Here's how the part is built. I have some questions about the finished solid (model axes, mm). Face numbers are marked on the shaded views. A direction names the side the tool comes from. Give positions to 0.01 mm unless a question says otherwise; leave off trailing zeros. Write each loop counter-clockwise with the first axis right and the second up, starting at its lowest first coordinate (ties: lowest second). Pieces come first, ordered by that corner, then holes. Notation, with made-up numbers: (7, 53.25) -> (21, 53.25) arc R31 cw to (21, 86.25) -> close; hole circle Ø4 at (48.5, 51). An arc over 180 degrees is marked (long way). Return JSON: item names as keys, results as strings.
Autodesk Inventor part; units mm, degrees
ref_plane "YZ Plane" through (0, 0, 0) normal (1, 0, 0) x (0, 1, 0)
ref_plane "XZ Plane" through (0, 0, 0) normal (0, 1, 0) x (-1, 0, 0)
ref_plane "XY Plane" through (0, 0, 0) normal (0, 0, 1) x (1, 0, 0)
sketch "Sketch1" plane through (0, 0, 0) normal (0, 0, 1) x (1, 0, 0)
  line L0 (9.6801, -14.008) -> (7.2052, -11.5331) construction
  line L1 (7.2052, -11.5331) -> (11.5893, -7.1491) construction
  line L2 (11.5893, -7.1491) -> (14.0642, -9.6239) construction
  line L3 (14.0642, -9.6239) -> (9.6801, -14.008) construction
  arc A0 (12.6369, -4.7496) -> (4.7496, -12.6369) centre (0, 0) ccw construction
  line L4 (10.9298, -3.0424) -> (12.6369, -4.7496) construction
  line L5 (11.6618, -4.6122) -> (10.9298, -3.0424) construction
  arc A1 (11.6618, -4.6122) -> (10.8551, -4.47) centre (11.2086, -4.8235) ccw construction
  line L6 (10.7915, -4.5335) -> (10.8551, -4.47) construction
  arc A2 (10.7915, -4.5335) -> (10.6527, -4.9738) centre (11.1451, -4.887) ccw construction
  line L7 (10.915, -6.4612) -> (10.6527, -4.9738) construction
  arc A3 (10.7761, -6.9016) -> (10.915, -6.4612) centre (10.4226, -6.548) ccw construction
  line L8 (6.9016, -10.7761) -> (10.7761, -6.9016) construction
  arc A4 (6.4612, -10.915) -> (6.9016, -10.7761) centre (6.548, -10.4226) ccw construction
  line L9 (6.4612, -10.915) -> (4.9738, -10.6527) construction
  arc A5 (4.9738, -10.6527) -> (4.5335, -10.7915) centre (4.887, -11.1451) ccw construction
  line L10 (4.5335, -10.7915) -> (4.47, -10.8551) construction
  arc A6 (4.47, -10.8551) -> (4.6122, -11.6618) centre (4.8235, -11.2086) ccw construction
  line L11 (4.6122, -11.6618) -> (3.0424, -10.9298) construction
  line L12 (3.0424, -10.9298) -> (4.7496, -12.6369) construction
  line L13 (-1.7167, -14.6498) -> (-1.7167, -17.5) construction
  line L14 (-1.7167, -17.5) -> (1.7167, -17.5) construction
  line L15 (1.7167, -14.6498) -> (1.7167, -17.5) construction
  arc A7 (1.7167, -14.6498) -> (6.9595, -13.0049) centre (0, 0) ccw construction
  arc A8 (6.9595, -13.0049) -> (8.2728, -15.1789) centre (8.2994, -13.6792) ccw construction
  line L16 (8.2728, -15.1789) -> (7.6816, -15.1684) construction
  arc A9 (8.5249, -17.8901) -> (7.6816, -15.1684) centre (7.655, -16.6682) ccw construction
  line L17 (8.5249, -17.8901) -> (13.5161, -14.3366) construction
  line L18 (13.5161, -14.3366) -> (13.5161, -12.2823) construction
  line L19 (13.5161, -12.2823) -> (14.6168, -12.2823) construction
  line L20 (14.6168, -12.2823) -> (14.6168, -1.9776) construction
  arc A10 (14.6168, -1.9776) -> (1.7167, 14.6498) centre (0, 0) ccw construction
  line L21 (1.7167, 14.6498) -> (1.7167, 17.5) construction
  line L22 (-1.7167, 17.5) -> (1.7167, 17.5) construction
  line L23 (-1.7167, 14.6498) -> (-1.7167, 17.5) construction
  arc A11 (-1.7167, 14.6498) -> (-14.2817, -3.6872) centre (0, 0) ccw construction
  line L24 (-14.2817, -3.6872) -> (-15.4135, -5.7935) construction
  arc A12 (-15.4135, -5.7935) -> (-14.5984, -8.502) centre (-13.6517, -6.7402) ccw construction
  line L25 (-14.5984, -8.502) -> (-9.6326, -11.1703) construction
  arc A13 (-9.6326, -11.1703) -> (-1.7167, -14.6498) centre (0, 0) ccw construction
  line L26 (-24.6, 24.6) -> (25.2, -25.2) construction
  line L27 (25.2, 24.6) -> (-24.6, -25.2) construction
  arc A14 (-1.7471, 10.1) -> (-9.6204, -3.5369) centre (0, 0) ccw
  circle A15 centre (0, 0) radius 10.1 construction
  line L28 (-1.7471, 10.1) -> (1.7471, 10.1)
  line L29 (-7.8733, -6.5631) -> (-9.6204, -3.5369)
  line L30 (9.6204, -3.5369) -> (7.8733, -6.5631)
  arc A16 (1.7471, 10.1) -> (-1.7471, 10.1) centre (0, 0) ccw
  arc A17 (9.6204, -3.5369) -> (1.7471, 10.1) centre (0, 0) ccw
  arc A18 (7.8733, -6.5631) -> (9.6204, -3.5369) centre (0, 0) ccw
  arc A19 (-7.8733, -6.5631) -> (7.8733, -6.5631) centre (0, 0) ccw
  arc A20 (-9.6204, -3.5369) -> (-7.8733, -6.5631) centre (0, 0) ccw
  arc A21 (10.7786, -4.5205) -> (10.6704, -4.6789) centre (11.1451, -4.887) ccw construction
  line L31 (10.7786, -4.5205) -> (10.8421, -4.457) construction
  arc A22 (11.7261, -4.7937) -> (10.8421, -4.457) centre (11.2086, -4.8235) ccw construction
  line L32 (11.7261, -4.7937) -> (10.8691, -2.9558) construction
  line L33 (10.8691, -2.9558) -> (12.6297, -4.7164) construction
  line L34 (4.7164, -12.6297) -> (2.9558, -10.8691) construction
  line L35 (2.9558, -10.8691) -> (4.4463, -11.5641) construction
  arc A23 (4.457, -10.8421) -> (4.4463, -11.5641) centre (4.8235, -11.2086) ccw construction
  line L36 (4.457, -10.8421) -> (4.5223, -10.7767) construction
  arc A24 (4.977, -10.6346) -> (4.6789, -10.6704) centre (4.887, -11.1451) ccw
  arc A25 (4.6789, -10.6704) -> (4.5223, -10.7767) centre (4.887, -11.1451) ccw construction
  arc A26 (10.6704, -4.6789) -> (10.6346, -4.977) centre (11.1451, -4.887) ccw
  circle A27 centre (0, 0) radius 12.65
  dimension "d4" = 20.2
  dimension "d6" = 20.5
  dimension "d9" = 360
  dimension "d28" = 25.3
extrude "Extrusion1" add sketch "Sketch1" against normal blind 5 contours A16 L28 | L29 A20 | A18 L30 | A27
sketch "Sketch3" plane through (0, 0, -5) normal (0, 0, -1) x (-1, 0, 0)
  arc A0 (-7.8733, -6.5631) -> (7.8733, -6.5631) centre (0, 0) ccw
  circle A1 centre (0, 0) radius 9
  circle A2 centre (0, 0) radius 11.5312
  circle A3 centre (0, 0) radius 12.65
  line L0 (9.6204, -3.5369) -> (7.8733, -6.5631)
  line L1 (-7.8733, -6.5631) -> (-9.6204, -3.5369)
  arc A4 (-1.7471, 10.1) -> (-9.6204, -3.5369) centre (0, 0) ccw
  line L2 (-1.7471, 10.1) -> (1.7471, 10.1)
  arc A5 (9.6204, -3.5369) -> (1.7471, 10.1) centre (0, 0) ccw
  dimension "d17" = 18
extrude "Extrusion3" add sketch "Sketch3" along normal blind 10 contours L1 A4 L2 A5 L0 A0 | A2 | A3
sketch "Sketch4" plane through (0, -10.7054, 0) normal (1, 0, 0) x (0, 0, -1)
  line L0 (15, 19.7054) -> (15, 1.7054)
  line L1 (5, 1.7054) -> (5, 19.7054)
  circle A0 centre (13, 10.7054) radius 1.4
  circle A1 centre (7, 10.7054) radius 1.4
  dimension "d24" = 2.8
  dimension "d25" = 2.8
  dimension "d26" = 6
  dimension "d27" = 2
extrude "Extrusion4" cut sketch "Sketch4" against normal through all
properties part number "20_focus_inlet_objective_mount_v8"
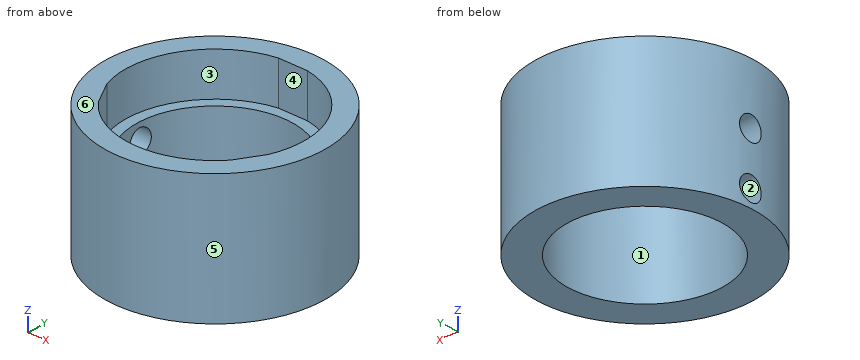
1. For pin 1 Ø1 at (x, y) = (-8, 4) entering from +Z; pin 2 Ø3 at (x, z) = (2.5, -10) entering from +Y; pin 3 Ø1 at (x, z) = (4, -2.5) entering from +Y, each with a flat end and sliding along its axis, tell me the tip position at first contact or that it passes through.
Taken from the geometry:
{"pin 1": "stops at z = -5", "pin 2": "stops at y = 12.61", "pin 3": "stops at y = 12.16"}
2. If I drill on line 1 (Z direction, x = -11.7, y = 0); line 2 (Z direction, x = -10.2, y = 0); line 3 (Y direction, x = 0, z = -8), over which ranges is the centre line in solid material (lowest first)? Write a range as [from, to].
Taken from the geometry:
{"line 1": "z = [-15, -14.4], [-11.6, -8.4], [-5.6, 0]", "line 2": "z = [-15, -14.4], [-11.6, -8.4], [-5.6, -5]", "line 3": "y = [-12.65, -9], [9, 12.65]"}
3. Suppose I cut it at A-A, the plane y = 0. List the corners of the cut face in (x, z) for me.
Taken from the geometry:
{"outline": "(-12.65, -15) -> (-9, -15) -> (-9, -14.4) -> (-12.65, -14.4) -> close; (-12.65, -11.6) -> (-9, -11.6) -> (-9, -8.4) -> (-12.65, -8.4) -> close; (-12.65, -5.6) -> (-9, -5.6) -> (-9, -5) -> (-10.25, -5) -> (-10.25, 0) -> (-12.65, 0) -> close; (9, -15) -> (12.65, -15) -> (12.65, 0) -> (10.25, 0) -> (10.25, -5) -> (9, -5) -> close"}
4. Suppose I cut it at D-D, the plane y = 6.5. List the corners of the cut face in (x, z) for me.
Taken from the geometry:
{"outline": "(-10.85, -15) -> (-6.22, -15) -> (-6.22, -5) -> (-7.93, -5) -> (-7.93, 0) -> (-10.85, 0) -> close; (6.22, -15) -> (10.85, -15) -> (10.85, 0) -> (7.93, 0) -> (7.93, -5) -> (6.22, -5) -> close"}
5. Suppose I cut it at C-C, the plane z = -1.25. List the corners of the cut face in (x, y) for me.
Taken from the geometry:
{"outline": "circle Ø25.3 at (0, 0); hole (-9.62, -3.54) -> (-7.87, -6.56) arc R10.25 ccw to (7.87, -6.56) -> (9.62, -3.54) arc R10.25 ccw to (1.75, 10.1) -> (-1.75, 10.1) arc R10.25 ccw to start"}
6. Which directions (+Z, -Z, +X, -X, +Y, -Y) give clear straight access to the entire face, cutting with the end or side of a thin tool? Please do the marked faces 1, 2 and 3.
Taken from the geometry:
{"face 1": "+Z, -Z", "face 2": "-X", "face 3": "+Z"}
7. If we mould it in two halves opening along X, with no side actions, what happens to the marked faces 4, 5 and 6? For each: released by +X, released by -X, zero draft, split by the parting line, or undercut.
Taken from the geometry:
{"face 4": "undercut", "face 5": "split by the parting line", "face 6": "zero draft"}
8. Suppose I cut it at B-B, the plane x = 0. List the corners of the cut face in (y, z) for me, and give its area (4 significant figures).
Taken from the geometry:
{"outline": "(-12.65, -15) -> (-9, -15) -> (-9, -5) -> (-10.25, -5) -> (-10.25, 0) -> (-12.65, 0) -> close; (9, -15) -> (12.65, -15) -> (12.65, 0) -> (10.1, 0) -> (10.1, -5) -> (9, -5) -> close", "area": "97.75 mm²"}
